```python
from build123d import *

# Parameters (mm, degrees)
F0_W      = 101.6
F0_H      = 101.6
F1_DEPTH  = 101.6
F2_R      = 44.45
F3_DEPTH  = 12.7
F4_R      = 31.75
F5_DEPTH  = 12.7
F6_R      = 19.05
F7_DEPTH  = 23.8125
F8_R      = 44.45
F8_R_2    = 31.75
F8_R_3    = 19.05
F9_DEPTH  = 12.7
F10_DEPTH = 25.4
F11_DEPTH = 49.2252
F12_R     = 19.05
F15_DEPTH = 49.2252
F13_R     = 19.05
F16_DEPTH = 49.2252
F13_R_2   = 31.75
F17_DEPTH = 25.4
F13_R_3   = 44.45
F18_DEPTH = 12.7
F14_R     = 19.05
F19_DEPTH = 49.1998
F14_R_2   = 31.75
F20_DEPTH = 25.4
F14_R_3   = 44.45
F21_DEPTH = 12.7
F12_R_2   = 31.75
F22_DEPTH = 25.4
F12_R_3   = 44.45
F23_DEPTH = 12.7


with BuildPart() as f1:
    # F0 (on Front) → F1 (new body)
    with BuildSketch(Plane.XZ):
        with Locations((-50.849611, 50.678841)):
            Rectangle(F0_W, F0_H)
    extrude(amount=F1_DEPTH)

    # F2 (on face) → F3 (cut)
    with BuildSketch(Plane.XZ.offset(101.6)):
        with Locations((-50.849611, 50.678841)):
            Circle(F2_R)
    extrude(amount=-F3_DEPTH, mode=Mode.SUBTRACT)

    # F4 (on face) → F5 (cut)
    with BuildSketch(Plane.XZ.offset(88.9)):
        with Locations((-50.849611, 50.678841)):
            Circle(F4_R)
    extrude(amount=-F5_DEPTH, mode=Mode.SUBTRACT)

    # F6 (on face) → F7 (cut)
    with BuildSketch(Plane.XZ.offset(76.2)):
        with Locations((-50.849611, 50.678841)):
            Circle(F6_R)
    extrude(amount=-F7_DEPTH, mode=Mode.SUBTRACT)

    # F8 (on face) → F9 (cut)
    with BuildSketch(Plane.XY.offset(101.478841)):
        with Locations((-50.849611, -50.8)):
            Circle(F8_R)
        with Locations((-50.849611, -50.8)):
            Circle(F8_R_2, mode=Mode.SUBTRACT)
        with Locations((-50.849611, -50.8)):
            Circle(F8_R_2)
        with Locations((-50.849611, -50.8)):
            Circle(F8_R_3, mode=Mode.SUBTRACT)
        with Locations((-50.849611, -50.8)):
            Circle(F8_R_3)
    extrude(amount=-F9_DEPTH, mode=Mode.SUBTRACT)

    # F8 (on face) → F10 (cut)
    with BuildSketch(Plane.XY.offset(101.478841)):
        with Locations((-50.849611, -50.8)):
            Circle(F8_R_2)
        with Locations((-50.849611, -50.8)):
            Circle(F8_R_3, mode=Mode.SUBTRACT)
        with Locations((-50.849611, -50.8)):
            Circle(F8_R_3)
    extrude(amount=-F10_DEPTH, mode=Mode.SUBTRACT)

    # F8 (on face) → F11 (cut)
    with BuildSketch(Plane.XY.offset(101.478841)):
        with Locations((-50.849611, -50.8)):
            Circle(F8_R_3)
    extrude(amount=-F11_DEPTH, mode=Mode.SUBTRACT)

    # F12 (on face) → F15 (cut)
    with BuildSketch(Plane.YZ.offset(-0.049611)):
        with Locations((-50.8, 50.678841)):
            Circle(F12_R)
    extrude(amount=-F15_DEPTH, mode=Mode.SUBTRACT)

    # F13 (on face) → F16 (cut)
    with BuildSketch(Plane(origin=(0, 0, 0), x_dir=(-1, 0, 0), z_dir=(0, 1, 0))):
        with Locations((50.849611, 50.678841)):
            Circle(F13_R)
    extrude(amount=-F16_DEPTH, mode=Mode.SUBTRACT)

    # F13 (on face) → F17 (cut)
    with BuildSketch(Plane(origin=(0, 0, 0), x_dir=(-1, 0, 0), z_dir=(0, 1, 0))):
        with Locations((50.849611, 50.678841)):
            Circle(F13_R_2)
        with Locations((50.849611, 50.678841)):
            Circle(F13_R, mode=Mode.SUBTRACT)
    extrude(amount=-F17_DEPTH, mode=Mode.SUBTRACT)

    # F13 (on face) → F18 (cut)
    with BuildSketch(Plane(origin=(0, 0, 0), x_dir=(-1, 0, 0), z_dir=(0, 1, 0))):
        with Locations((50.849611, 50.678841)):
            Circle(F13_R_3)
        with Locations((50.849611, 50.678841)):
            Circle(F13_R_2, mode=Mode.SUBTRACT)
    extrude(amount=-F18_DEPTH, mode=Mode.SUBTRACT)

    # F14 (on face) → F19 (cut)
    with BuildSketch(Plane(origin=(-101.649611, 0, 0), x_dir=(0, -1, 0), z_dir=(-1, 0, 0))):
        with Locations((50.8, 50.678841)):
            Circle(F14_R)
    extrude(amount=-F19_DEPTH, mode=Mode.SUBTRACT)

    # F14 (on face) → F20 (cut)
    with BuildSketch(Plane(origin=(-101.649611, 0, 0), x_dir=(0, -1, 0), z_dir=(-1, 0, 0))):
        with Locations((50.8, 50.678841)):
            Circle(F14_R_2)
        with Locations((50.8, 50.678841)):
            Circle(F14_R, mode=Mode.SUBTRACT)
    extrude(amount=-F20_DEPTH, mode=Mode.SUBTRACT)

    # F14 (on face) → F21 (cut)
    with BuildSketch(Plane(origin=(-101.649611, 0, 0), x_dir=(0, -1, 0), z_dir=(-1, 0, 0))):
        with Locations((50.8, 50.678841)):
            Circle(F14_R_3)
        with Locations((50.8, 50.678841)):
            Circle(F14_R_2, mode=Mode.SUBTRACT)
    extrude(amount=-F21_DEPTH, mode=Mode.SUBTRACT)

    # F12 (on face) → F22 (cut)
    with BuildSketch(Plane.YZ.offset(-0.049611)):
        with Locations((-50.8, 50.678841)):
            Circle(F12_R_2)
        with Locations((-50.8, 50.678841)):
            Circle(F12_R, mode=Mode.SUBTRACT)
    extrude(amount=-F22_DEPTH, mode=Mode.SUBTRACT)

    # F12 (on face) → F23 (cut)
    with BuildSketch(Plane.YZ.offset(-0.049611)):
        with Locations((-50.8, 50.678841)):
            Circle(F12_R_3)
        with Locations((-50.8, 50.678841)):
            Circle(F12_R_2, mode=Mode.SUBTRACT)
    extrude(amount=-F23_DEPTH, mode=Mode.SUBTRACT)


solid = f1.part
```
Source: CAD feature listing. Evaluate the final solid. Frame: model axes, mm. A direction names the side the tool comes from. Round coordinates to 2 decimals unless told otherwise and drop trailing zeros. Loops run counter-clockwise (first coordinate to the right, second up) from the corner with the lowest first, then second, coordinate; pieces in that order, holes last. Notation, with made-up numbers: M -34.5,41 L -6.5,41 A12 cw -6.5,58 Z; hole C 11.25,33 d4. An arc over 180 degrees is marked long. Use a Markdown table: item, result. Add a question column.
1. Cut plane A-A, the plane x = -30. State how many separate pieces and enclosed holes the cut face has, and give its area (3 significant figures).
2. Cut plane B-B, the plane y = -79. Output: boundary loops of the cut face in (x, z).
3. Set-up query: faces 4 (the cylindrical face through (-60.485, -96.75, 7.286)), 5 (the flat face through (-76.25, -39, 35)), 6 (the cylindrical face through (-17.6, -57.683, 19.684)). Return all of +Z, -Z, +X, -X, +Y, -Y with unobstructed straight access to the full face (end or side cutting, diameter ignored); none if empty.
4. Cut plane C-C, the plane x = -79. Output: boundary loops of the cut face in (y, z), and give its area (3 significant figures).
5. Contact query for flat-ended pins moving along their axis: pin 1 (12 mm diameter, centred on x = -58.5, z = 68, fed in from +Y); pin 2 (3.5 mm diameter, centred on x = -50.5, z = 45.5, fed in from +Y); pin 3 (23 mm diameter, centred on x = -50.85, z = 50.68, fed in from -Y). Output: stop coordinate, or through.
6. Ray query, line 1 along Y through (x, z) = (-73, 30); line 2 along X through (y, z) = (-63, 35.5); line 3 along Z through (x, y) = (-74, -24). Return the intervals inside material, ascending. Write a range as [from, to].
7. Pull-direction query (Y, two-part tool) for faces 1 (the cylindrical face through (-69.81, -46.67, 32.08)), 2 (the flat face through (-52.45, -51, 42)), 3 (the flat face through (-6, 0, 51)); classes: +Y half, -Y half, draft (parallel to the pull), parting line (faces both ways), or undercut.
Solution:
| question | item | result |
|---|---|---|
| 1 | separate pieces | 3 |
| 1 | enclosed holes | 1 |
| 1 | area | 4,370 mm2 |
| 2 | outline | M -101.65,-0.12 L -0.05,-0.12 L -0.05,16.32 L -12.75,16.32 L -12.75,36.09 L -22.65,36.09 A31.75 cw -79.05,36.09 L -88.95,36.09 L -88.95,16.32 L -101.65,16.32 Z; M -101.65,85.04 L -88.95,85.04 L -88.95,65.27 L -79.05,65.27 A31.75 cw -65.44,78.88 L -65.44,88.78 L -85.21,88.78 L -85.21,101.48 L -101.65,101.48 Z; M -36.26,78.88 A31.75 cw -22.65,65.27 L -12.75,65.27 L -12.75,85.04 L -0.05,85.04 L -0.05,101.48 L -16.49,101.48 L -16.49,88.78 L -36.26,88.78 Z |
| 3 | face 4 | -Y |
| 3 | face 5 | -X |
| 3 | face 6 | +X |
| 4 | outline | M -101.6,-0.12 L 0,-0.12 L 0,16.28 L -12.7,16.28 L -12.7,35.99 L -22.65,35.99 A31.75 cw -78.95,35.99 L -88.9,35.99 L -88.9,16.28 L -101.6,16.28 Z; M -101.6,85.08 L -88.9,85.08 L -88.9,65.36 L -78.95,65.36 A31.75 cw -65.48,78.83 L -65.48,88.78 L -85.2,88.78 L -85.2,101.48 L -101.6,101.48 Z; M -36.12,78.83 A31.75 cw -22.65,65.36 L -12.7,65.36 L -12.7,85.08 L 0,85.08 L 0,101.48 L -16.4,101.48 L -16.4,88.78 L -36.12,88.78 Z |
| 4 | area | 3,870 mm2 |
| 5 | pin 1 | stops at y = -25.4 |
| 5 | pin 2 | stops at y = -49.23 |
| 5 | pin 3 | stops at y = -52.39 |
| 6 | line 1 | y = [-76.2, -25.4] |
| 6 | line 2 | x = [-76.25, -62.36], [-39.34, -25.45] |
| 6 | line 3 | z = [-0.12, 28.95], [72.41, 88.78] |
| 7 | face 1 | undercut |
| 7 | face 2 | draft |
| 7 | face 3 | +Y half |
